Part model, mm, in its own coordinate system. A direction names the side the tool comes from. Coordinates: 2 decimals unless noted, no trailing zeros. Write each loop counter-clockwise with the first axis right and the second up, starting at its lowest first coordinate (ties: lowest second). Pieces come first, ordered by that corner, then holes. Notation, with made-up numbers: (1, 10) -> (11, 10) arc R22 cw to (11, 27) -> close; hole circle Ø7 at (-19.75, 41.25). An arc over 180 degrees is marked (long way). Write item = value, one per line.
from build123d import *

# Parameters (mm, degrees)
SKETCH1_W             = 66
SKETCH1_H             = 140
SKETCH1_R             = 3.25
SKETCH1_W_2           = 53
SKETCH1_H_2           = 81
BOSS_EXTRUDE1_DEPTH   = 3
FILLET1_R             = 2
M4X0_7_TAPPED_HOLE1_D = 3.3
M3X0_5_TAPPED_HOLE1_D = 2.5


with BuildPart() as part:
    # Sketch1 → Boss-Extrude1 (new body)
    with BuildSketch(Plane.XY):
        with Locations((22.144812637, -44.667286245)):
            Rectangle(SKETCH1_W, SKETCH1_H)
        with Locations((4.644812637, -99.667286245)):
            Circle(SKETCH1_R, mode=Mode.SUBTRACT)
        with Locations((39.644812637, -99.667286245)):
            Circle(SKETCH1_R, mode=Mode.SUBTRACT)
        with Locations((22.144812637, -29.867286245)):
            Rectangle(SKETCH1_W_2, SKETCH1_H_2, mode=Mode.SUBTRACT)
    extrude(amount=BOSS_EXTRUDE1_DEPTH)

    # Fillet1
    fillet1_edges = [part.edges().sort_by_distance(p)[0] for p in [
        (-10.855187363, 25.332713755, 1.5),
        (55.144812637, 25.332713755, 1.5),
        (55.144812637, -114.667286245, 1.5),
        (-10.855187363, -114.667286245, 1.5),
    ]]
    fillet(fillet1_edges, radius=FILLET1_R)

    # M4x0.7 Tapped Hole1 (through all)
    with Locations(Plane.XY.offset(3)):
        with Locations((22.144812637, 15.132713755), (22.144812637, -74.867286245)):
            Hole(M4X0_7_TAPPED_HOLE1_D / 2)

    # M3x0.5 Tapped Hole1 (through all)
    with Locations(Plane.XY.offset(3)):
        with Locations((48.644812637, 15.632713755), (-4.355187363, -75.367286245)):
            Hole(M3X0_5_TAPPED_HOLE1_D / 2)


solid = part.part
Q1. Saw through at D-D on y = -101.5. Give the cut face in (x, z).
Model answer:
outline = (-10.86, 0) -> (1.96, 0) -> (1.96, 3) -> (-10.86, 3) -> close; (7.33, 0) -> (36.96, 0) -> (36.96, 3) -> (7.33, 3) -> close; (42.33, 0) -> (55.14, 0) -> (55.14, 3) -> (42.33, 3) -> close
Q2. Saw through at B-B on y = -2. Give the cut face in (x, z), and give its area (3 significant figures).
Model answer:
outline = (-10.86, 0) -> (-4.36, 0) -> (-4.36, 3) -> (-10.86, 3) -> close; (48.64, 0) -> (55.14, 0) -> (55.14, 3) -> (48.64, 3) -> close
area = 39.0 mm²
Q3. Probe line 1 (Y direction, x = 39.5, z = 1.4); line 2 (X direction, y = -49, z = 1.9); line 3 (Y direction, x = 45, z = 2.6). List the from-to ranges inside material, lowest first. Write a range as from..to.
Model answer:
line_1 = -114.67..-102.91, -96.42..-70.37, 10.63..25.33
line_2 = -10.86..-4.36, 48.64..55.14
line_3 = -114.67..-70.37, 10.63..25.33
Q4. Mould opens along X. For faces 3 (the face through (22, 10.633, 1)), 4 (the face through (22, -114.667, 1)), 5 (the face through (-10.855, -46, 1)) say: released by +X, released by -X, zero draft, split by the parting line, or undercut.
Model answer:
face_3 = undercut
face_4 = zero draft
face_5 = released by -X
Q5. Saw through at A-A on x = 28. Give the cut face in (y, z).
Model answer:
outline = (-114.67, 0) -> (-70.37, 0) -> (-70.37, 3) -> (-114.67, 3) -> close; (10.63, 0) -> (25.33, 0) -> (25.33, 3) -> (10.63, 3) -> close
Q6. Which spindle directions (+Z, -Z, +X, -X, +Y, -Y) get a long thin tool onto all of the face, cutting with end or side? Do faces 1 (the face through (-4.355, -30, 1)), 2 (the face through (55.145, -46, 1)). Say none if no direction does.
Model answer:
face_1 = +Z, -Z
face_2 = +Z, -Z, +X, +Y, -Y
Q7. Saw through at C-C on x = 40.5. Give the cut face in (y, z).
Model answer:
outline = (-114.67, 0) -> (-102.8, 0) -> (-102.8, 3) -> (-114.67, 3) -> close; (-96.53, 0) -> (-70.37, 0) -> (-70.37, 3) -> (-96.53, 3) -> close; (10.63, 0) -> (25.33, 0) -> (25.33, 3) -> (10.63, 3) -> close
